The listing builds one solid part. Answer for the finished solid, in the listing's coordinates (mm). A direction names the side the tool comes from. Coordinates: 2 decimals unless noted, no trailing zeros. Order: outer loops, then holes, each group sorted by start corner. A loop starts at its lowest first (then second) coordinate and runs counter-clockwise, first axis right, second up.
Autodesk Inventor part; units mm, degrees
ref_plane "YZ Plane" through (0, 0, 0) normal (1, 0, 0) x (0, 1, 0)
ref_plane "XZ Plane" through (0, 0, 0) normal (0, 1, 0) x (-1, 0, 0)
ref_plane "XY Plane" through (0, 0, 0) normal (0, 0, 1) x (1, 0, 0)
sketch "Sketch1" plane through (0, 0, 0) normal (0, 1, 0) x (-1, 0, 0)
  circle A0 centre (0, 0) radius 70
  dimension "d0" = 140
extrude "Extrusion1" add sketch "Sketch1" along normal blind 30
sketch "Sketch2" plane through (0, 30, 0) normal (0, 1, 0) x (1, 0, 0)
  point P0 (0, 0)
fillet "Fillet1" radius 5.175 1 edges at (70, 30, 0)
sketch "Sketch3" plane through (0, 0, 0) normal (0, -1, 0) x (1, 0, 0)
  circle A0 centre (0, 0) radius 65
  dimension "d4" = 130
extrude "Extrusion2" cut sketch "Sketch3" against normal blind 25
sketch "Sketch5" plane through (0, 25, 0) normal (0, -1, 0) x (1, 0, 0)
  line L0 (-7, 0) -> (7, 0) construction
  line L1 (-7, -3) -> (7, -3)
  line L2 (7, 3) -> (-7, 3)
  arc A0 (-7, 3) -> (-7, -3) centre (-7, 0) ccw
  arc A1 (7, -3) -> (7, 3) centre (7, 0) ccw
  point P0 (0, 0)
  dimension "d11" = 7
  dimension "d12" = 6
extrude "Extrusion4" add sketch "Sketch5" along normal blind 20
sketch "Sketch6" plane through (0, 5, 0) normal (0, -1, 0) x (1, 0, 0)
  line L0 (-5, 0) -> (5, 0) construction
  line L1 (-5, -1.5) -> (5, -1.5)
  line L2 (5, 1.5) -> (-5, 1.5)
  arc A0 (-5, 1.5) -> (-5, -1.5) centre (-5, 0) ccw
  arc A1 (5, -1.5) -> (5, 1.5) centre (5, 0) ccw
  point P0 (0, 0)
  dimension "d15" = 5
  dimension "d16" = 3
extrude "Extrusion5" cut sketch "Sketch6" against normal blind 20
properties part number "Drehplatform_prototyp"
(1) Find section B-B on x = 0. Determine the outline of the cut face in (y, z) (3 decimals), then the cut area to 3 significant figures.
(2) Find section A-A on y = 16.5. Determine the outline of the cut face in (x, z), then the cut area to 3 significant figures.
(3) Find the intervals of material crossed by probe 1 along Z at (x, y) = (0, 9.25); probe 2 along X at (y, z) = (16.75, -2.5); probe 3 along X at (y, z) = (17.5, 1), in increasing order.
(4) Given pin 1 Ø5 at (x, z) = (54.5, 0) entering from -Y; pin 2 Ø7 at (x, y) = (2, 18) entering from +Z; pin 3 Ø6 at (y, z) = (26, 10.5) entering from +X, each flat-ended and moving along its own axis, determine where each tip first touches the part or whether it passes through.
(5) The mould has two halves that part along Z. Classify faces 1 (the flat face through (0, 15, 3)), 2 (the flat face through (-61.9, 0, -20.4)), 3 (the cylindrical face through (55.55, 12.239, 42.594)): pulls with the +Z half, pulls with the -Z half, needs draft (parallel to the pull), parting line crosses it, or undercut.
(6) A tool of negligible diameter and unlimited length cuts with its end or side. For faces 4 (the flat face through (1, 30, 1)), 5 (the flat face through (0, 15, -1.5)), from which of +Z, -Z, +X, -X, +Y, -Y can it reach the whole face along a straight path? Write none if from no direction.
Resolved:
1. outline: (0, -70) - (24.825, -70) arc R5.175 ccw to (30, -64.825) - (30, 64.825) arc R5.175 ccw to (24.825, 70) - (0, 70) - (0, 65) - (25, 65) - (25, 3) - (5, 3) - (5, 1.5) - (25, 1.5) - (25, -1.5) - (5, -1.5) - (5, -3) - (25, -3) - (25, -65) - (0, -65) - close
1. area: 999 mm2
2. outline: circle Ø140 at (0, 0); (-7, -3) - (7, -3) arc R3 ccw to (7, 3) - (-7, 3) arc R3 ccw to start; hole circle Ø130 at (0, 0); hole (-5, -1.5) - (5, -1.5) arc R1.5 ccw to (5, 1.5) - (-5, 1.5) arc R1.5 ccw to start
2. area: 2,200 mm2
3. probe 1: z = -70 to -65, -3 to -1.5, 1.5 to 3, 65 to 70
3. probe 2: x = -69.96 to -64.95, -8.66 to 8.66, 64.95 to 69.96
3. probe 3: x = -69.99 to -64.99, -9.83 to -6.12, 6.12 to 9.83, 64.99 to 69.99
4. pin 1: stops at y = 25
4. pin 2: stops at z = 70
4. pin 3: stops at x = 69.58
5. face 1: undercut
5. face 2: needs draft
5. face 3: parting line crosses it
6. face 4: +Z, -Z, +X, -X, +Y
6. face 5: -Y
